Can you work these out from the model? Positions are in its coordinate system, mm. Coordinates: 2 decimals unless noted, no trailing zeros. Order: outer loops, then holes, each group sorted by start corner. A loop starts at its lowest first (then second) coordinate and runs counter-clockwise, first axis right, second up. Notation, with made-up numbers: (-5, 72.25) -> (31, 72.25) arc R29 ccw to (31, 103.25) -> close; hole circle Ø6 at (43, 2). An arc over 180 degrees is marked (long way). Answer as a JSON object with one key per item and string values. Group by question number.
(1) For pin 1 (5 mm diameter, centred on x = 40, y = 0, fed in from +Z), with a flat end and sliding along its axis, tell me the tip position at first contact or that it passes through.
(2) I want a section at D-D, the plane y = 3.75. List the corners of the cut face in (x, z) for me, plus the area to 3 significant figures.
(3) I want a section at B-B, the plane z = 0.25. State how many separate pieces and enclosed holes the cut face has, plus the area to 3 significant figures.
(4) I need wall thicknesses on line 1 (Y direction, x = 40, z = 0.3); line 2 (Y direction, x = 48.5, z = 0.65); line 3 (X direction, y = -4.25, z = 0.65). Which ranges of each line are inside material? Lowest first, please.
(5) I want a section at A-A, the plane x = 80. List the corners of the cut face in (y, z) for me, plus the area to 3 significant figures.
from build123d import *

# Parameters (mm, degrees)
SKETCH_R  = 2.1
PAD_DEPTH = 1


with BuildPart() as part:
    # Sketch → Pad (new body)
    with BuildSketch(Plane.XY):
        with BuildLine():
            ThreePointArc((0, 5), (-5, 0), (0, -5))
            Line((0, -5), (90, -5))
            ThreePointArc((90, -5), (95, 0), (90, 5))
            Line((0, 5), (90, 5))
        make_face()
        Circle(SKETCH_R, mode=Mode.SUBTRACT)
        with Locations((10, 0)):
            Circle(SKETCH_R, mode=Mode.SUBTRACT)
        with Locations((20, 0)):
            Circle(SKETCH_R, mode=Mode.SUBTRACT)
        with Locations((30, 0)):
            Circle(SKETCH_R, mode=Mode.SUBTRACT)
        with Locations((40, 0)):
            Circle(SKETCH_R, mode=Mode.SUBTRACT)
        with Locations((50, 0)):
            Circle(SKETCH_R, mode=Mode.SUBTRACT)
        with Locations((60, 0)):
            Circle(SKETCH_R, mode=Mode.SUBTRACT)
        with Locations((70, 0)):
            Circle(SKETCH_R, mode=Mode.SUBTRACT)
        with Locations((80, 0)):
            Circle(SKETCH_R, mode=Mode.SUBTRACT)
        with Locations((90, 0)):
            Circle(SKETCH_R, mode=Mode.SUBTRACT)
    extrude(amount=PAD_DEPTH)


solid = part.part
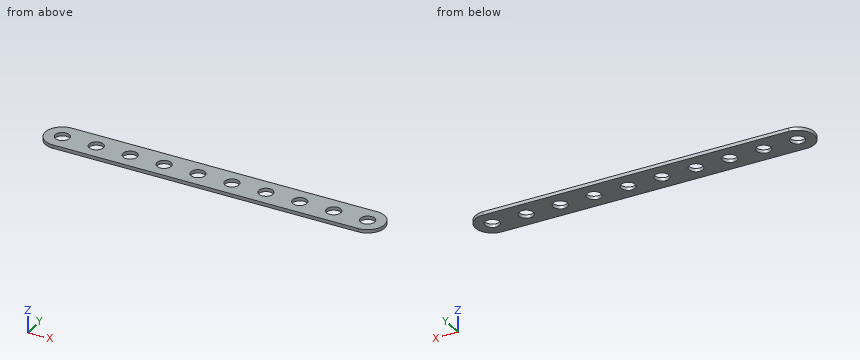
Computed values:
{
 "1": {"pin 1": "stops at z = 1"},
 "2": {"outline": "(-3.31, 0) -> (93.31, 0) -> (93.31, 1) -> (-3.31, 1) -> close", "area": "96.6 mm2"},
 "3": {"separate pieces": "1", "enclosed holes": "10", "area": "840 mm2"},
 "4": {"line 1": "y = -5 to -2.1, 2.1 to 5", "line 2": "y = -5 to -1.47, 1.47 to 5", "line 3": "x = -2.63 to 92.63"},
 "5": {"outline": "(-5, 0) -> (-2.1, 0) -> (-2.1, 1) -> (-5, 1) -> close; (2.1, 0) -> (5, 0) -> (5, 1) -> (2.1, 1) -> close", "area": "5.80 mm2"}
}
